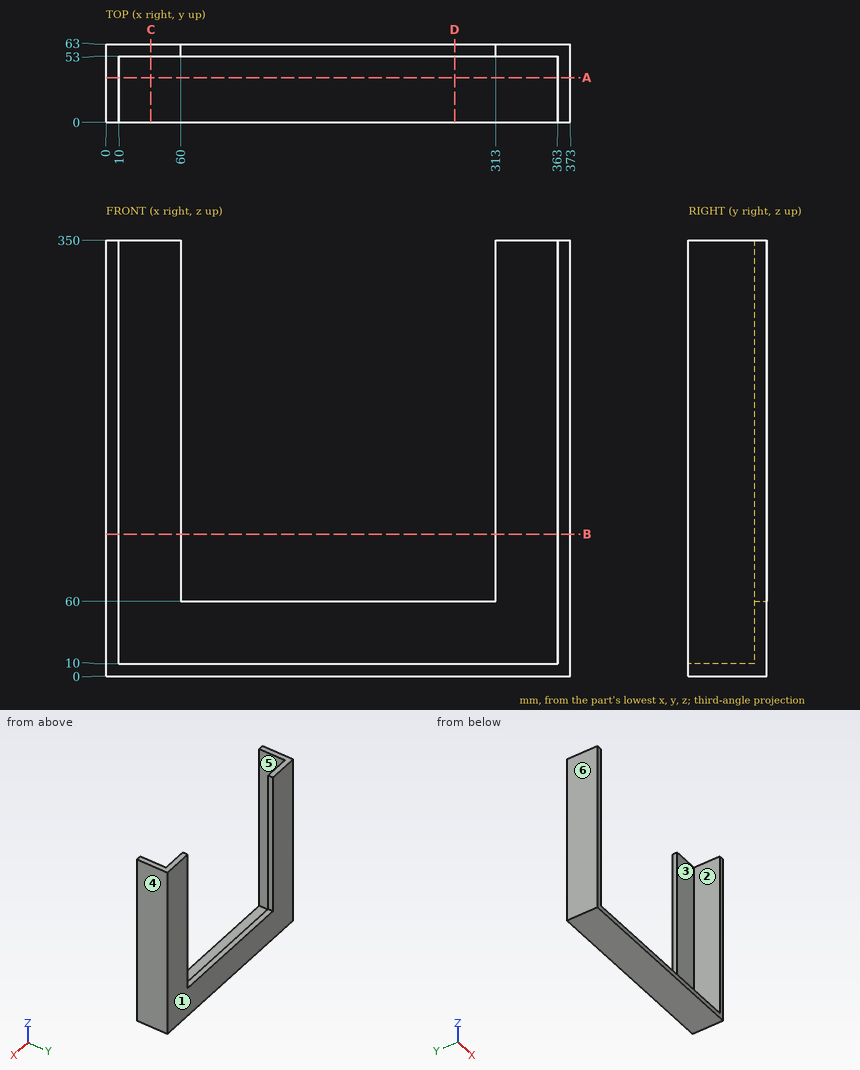
Geometry: see drawing. Coordinates: mm, zero at the bounding-box minimum. A direction names the side the tool comes from. Give positions to 0.01 mm unless a question says otherwise; leave off trailing zeros. Loops run counter-clockwise (first coordinate to the right, second up) from the corner with the lowest first, then second, coordinate; pieces in that order, holes last. Notation, with made-up numbers: (6.5, 26) - (27.5, 26) arc R12 ccw to (27.5, 33) - close; hole circle Ø9 at (34, -22.5). An arc over 180 degrees is marked (long way). One line per question, with ' | ' between items. Start each with the question number.
(1) Pull-direction query (X, two-part tool) for the marked faces 1, 2, 3 and 4; classes: released by +X, released by -X, zero draft, split by the parting line, or undercut.
(2) Ray query, line 1 (X direction, y = 44, z = 318); line 2 (Z direction, x = 175, y = 44.5); line 3 (Y direction, x = 31.5, z = 260). Return the intervals inside material, ascending. Write a range as from..to.
(3) Section query D-D on x = 280. Return loops of the section in (y, z), then the cut area to 3 significant figures.
(4) Contact query for flat-ended pins moving along their axis: pin 1 (11 mm diameter, centred on x = 182.5, y = 60, fed in from +Z); pin 2 (12 mm diameter, centred on x = 41.5, y = 12, fed in from +Z). Output: stop coordinate, or through.
(5) Section query C-C on x = 36. Return loops of the section in (y, z), then the cut area to 3 significant figures.
(6) Section query A-A on y = 36. Return loops of the section in (x, z), then the cut area to 3 significant figures.
(7) Section query B-B on z = 114. Return loops of the section in (x, y), then the cut area to 3 significant figures.
(8) Reachability of the marked faces 5 and 6 from +Z, -Z, +X, -X, +Y, -Y: full face, straight path, thin tool, end or side. Return the list, or none.
The answers:
1) face 1: zero draft | face 2: undercut | face 3: undercut | face 4: released by +X
2) line 1: 0..10, 363..373 | line 2: 0..10 | line 3: 53..63
3) outline: (0, 0) - (63, 0) - (63, 60) - (53, 60) - (53, 10) - (0, 10) - close | area: 1,130 mm2
4) pin 1: z = 60 | pin 2: z = 10
5) outline: (0, 0) - (63, 0) - (63, 350) - (53, 350) - (53, 10) - (0, 10) - close | area: 4,030 mm2
6) outline: (0, 0) - (373, 0) - (373, 350) - (363, 350) - (363, 10) - (10, 10) - (10, 350) - (0, 350) - close | area: 10,500 mm2
7) outline: (0, 0) - (10, 0) - (10, 53) - (60, 53) - (60, 63) - (0, 63) - close; (313, 53) - (363, 53) - (363, 0) - (373, 0) - (373, 63) - (313, 63) - close | area: 2,260 mm2
8) face 5: +Z, -Y | face 6: +Z, -Z, -X, +Y, -Y
